Design review of the part built by this model. Coordinates are the model's own, in mm. Face numbers are marked on the shaded views. Coordinates: 2 decimals unless noted, no trailing zeros. Write each loop counter-clockwise with the first axis right and the second up, starting at its lowest first coordinate (ties: lowest second). Pieces come first, ordered by that corner, then holes. Notation, with made-up numbers: (69.5, 42.5) -> (104.5, 42.5) arc R20 cw to (104.5, 65.5) -> close; hole circle Ø10 at (81, 40). An arc over 180 degrees is marked (long way). Return JSON: item names as keys, results as strings. Group by question number.
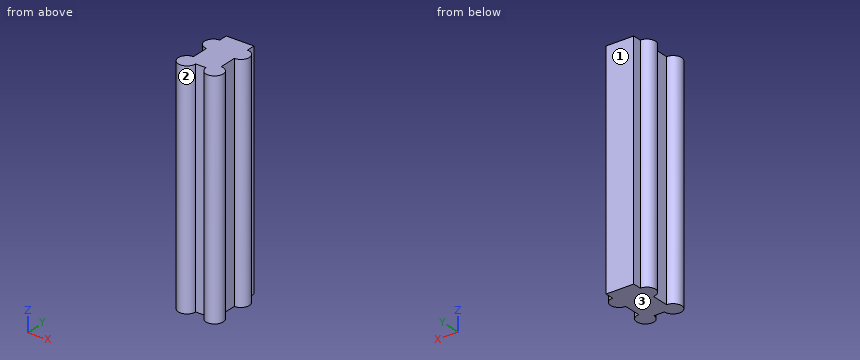
from build123d import *
from build123d.topology import SkipClean

# Parameters (mm, degrees)
SKETCH_1_R      = 5
SKETCH_1_W      = 16
SKETCH_1_H      = 30
EXTRUDE_1_DEPTH = 65


with BuildPart() as part:
    # Эскиз1 → Бобышка-Вытянуть1 (new, symmetric)
    with SkipClean():  # the faces are left unmerged after this step: merging them gives an invalid solid
        with BuildSketch(Plane(origin=(0, 0, 0), x_dir=(1, 0, 0), z_dir=(0, 0, -1))):
            with BuildLine():
                ThreePointArc((-8, 0), (-13, -5), (-8, -10))
                Line((-8, -10), (-8, 0))
            make_face()
            with BuildLine():
                Line((-8, 0), (-8, -10))
                ThreePointArc((-8, -10), (-4.464466094, -8.535533906), (-3, -5))
                ThreePointArc((-3, -5), (-4.464466094, -1.464466094), (-8, 0))
            make_face()
            with Locations((8, 15)):
                Circle(SKETCH_1_R)
            with Locations((8, -5)):
                Circle(SKETCH_1_R)
            with Locations((-8, -5)):
                Circle(SKETCH_1_R)
            with Locations((-8, 15)):
                Circle(SKETCH_1_R)
            Rectangle(SKETCH_1_W, SKETCH_1_H)
            with BuildLine():
                ThreePointArc((-3, 15), (-11.535533906, 18.535533906), (-8, 10))
                Line((-8, 10), (-8, 15))
                Line((-8, 15), (-3, 15))
            make_face()
            with BuildLine():
                Line((-8, 15), (-8, 10))
                ThreePointArc((-8, 10), (-4.464466094, 11.464466094), (-3, 15))
                Line((-3, 15), (-8, 15))
            make_face()
            with BuildLine():
                ThreePointArc((3, 15), (4.464466094, 11.464466094), (8, 10))
                Line((8, 10), (8, 15))
                Line((8, 15), (3, 15))
            make_face()
            with BuildLine():
                Line((8, 15), (8, 10))
                ThreePointArc((8, 10), (11.535533906, 11.464466094), (13, 15))
                ThreePointArc((13, 15), (8, 20), (3, 15))
                Line((3, 15), (8, 15))
            make_face()
            with BuildLine():
                ThreePointArc((8, 0), (3, -5), (8, -10))
                Line((8, -10), (8, 0))
            make_face()
            with BuildLine():
                Line((8, 0), (8, -10))
                ThreePointArc((8, -10), (11.535533906, -8.535533906), (13, -5))
                ThreePointArc((13, -5), (11.535533906, -1.464466094), (8, 0))
            make_face()
        extrude(amount=EXTRUDE_1_DEPTH, both=True)


solid = part.part
Q1. We need section C-C on x = 0.5. Write out the cut boundary in (y, z).
Q2. The part is to be moulded in two halves that separate along Y. For the marked faces 1, 2 and 3, say which applies: +Y half, -Y half, draft (parallel to the pull), parting line (faces both ways), or undercut.
Q3. We need section D-D on y = 12.5. Write out the cut boundary in (x, z), plus the area to 3 significant figures.
Q4. We need section B-B on z = -53. Write out the cut boundary in (x, y), plus the area to 3 significant figures.
Q5. Wall thickness on L1, parallel to X at y = -1.5, z = -34; L2, parallel to Y at x = 1.5, z = 53.5; L3, parallel to Y at x = -9.25, z = 48.5: over which ranges is each line inside the solid? List them lowest first.
Q6. For P1, Ø4, axis at y = 2.5, z = 47.5, coming from the +X side; P2, Ø5, axis at y = -5, z = 3.5, coming from the +X side; P3, Ø3, axis at y = -4.5, z = 0.5, coming from the -X side, all flat-tipped, find the tip position at first contact; note any pin that passes through.
Q7. We need section A-A on x = -11. Write out the cut boundary in (y, z).
Findings below:
{
 "1": {"outline": "(-15, -65) -> (15, -65) -> (15, 65) -> (-15, 65) -> close"},
 "2": {"face 1": "+Y half", "face 2": "undercut", "face 3": "draft"},
 "3": {"outline": "(-8, -65) -> (8, -65) -> (8, 65) -> (-8, 65) -> close", "area": "2,080 mm^2"},
 "4": {"outline": "(-8, -10) arc R5 ccw (long way) to (-3, -15) -> (3, -15) arc R5 ccw (long way) to (8, -10) -> (8, 0) arc R5 ccw to (8, 10) -> (8, 15) -> (-8, 15) -> (-8, 10) arc R5 ccw to (-8, 0) -> close", "area": "676 mm^2"},
 "5": {"L1": "x = -8 to 8", "L2": "y = -15 to 15", "L3": "y = -19.84 to -10.16, 0.16 to 9.84"},
 "6": {"P1": "stops at x = 12.97", "P2": "stops at x = 8", "P3": "stops at x = -8"},
 "7": {"outline": "(-19, -65) -> (-11, -65) -> (-11, 65) -> (-19, 65) -> close; (1, -65) -> (9, -65) -> (9, 65) -> (1, 65) -> close"}
}
